Source: CAD feature listing. Evaluate the final solid. Frame: model axes, mm. Face numbers are marked on the shaded views. A direction names the side the tool comes from. Give positions to 0.01 mm unless a question says otherwise; leave off trailing zeros. Order: outer loops, then holes, each group sorted by start corner. A loop starts at its lowest first (then second) coordinate and runs counter-clockwise, first axis right, second up.
from build123d import *

# Parameters (mm, degrees)
F1_DEPTH = 7.62
F3_R     = 1.651
F4_DEPTH = 25.4
F5_R     = 3.175
F6_DEPTH = 3.81
F7_W     = 55.88
F7_H     = 9.525
F8_DEPTH = 2.54


with BuildPart() as f1:
    # F0 (on Right) → F1 (new body, symmetric)
    with BuildSketch(Plane.YZ):
        Polygon((0, 0), (0, -9.8425), (27.94, -9.8425), (27.94, 9.525), (20.447, 9.525), (20.447, 0), align=None)
    extrude(amount=F1_DEPTH, both=True)

    # F2: F1 across plane


with BuildPart() as f1_1:
    add(f1.part)
    add(f1.part.mirror(Plane.XZ))

    # F3 (on face) → F4 (cut)
    with BuildSketch(Plane.YZ.offset(7.62)):
        with Locations((-24.257, 4.445)):
            Circle(F3_R)
        with Locations((24.257, 4.445)):
            Circle(F3_R)
    extrude(amount=-F4_DEPTH, mode=Mode.SUBTRACT)

    # F5 (on face) → F6 (cut)
    with BuildSketch(Plane(origin=(0, 0, -9.8425), x_dir=(1, 0, 0), z_dir=(0, 0, -1))):
        Circle(F5_R)
    extrude(amount=-F6_DEPTH, mode=Mode.SUBTRACT)

    # F7 (on face) → F8 (cut)
    with BuildSketch(Plane.YZ.offset(7.62)):
        with Locations((0, 4.7625)):
            Rectangle(F7_W, F7_H)
    extrude(amount=-F8_DEPTH, mode=Mode.SUBTRACT)


solid = f1_1.part
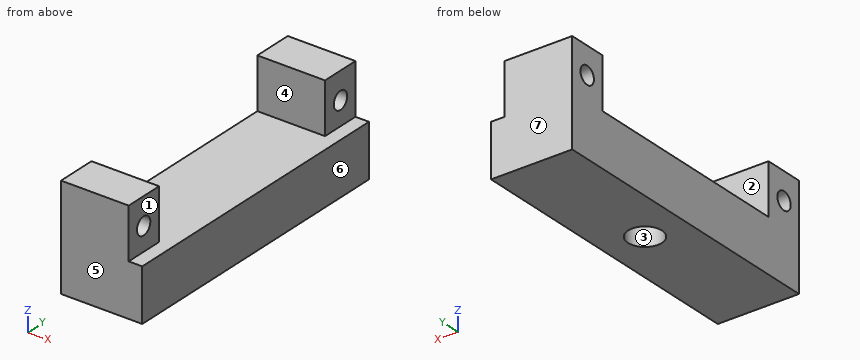
1) Ray query, L1, parallel to X at y = 0, z = -7.4 (3 decimals); L2, parallel to Y at x = -0.5, z = 7.5; L3, parallel to Y at x = -4, z = 3. Return the intervals inside material, ascending.
Checks:
L1: x = -7.62 to -3.175, 3.175 to 7.62
L2: y = -27.94 to -20.45, 20.45 to 27.94
L3: y = -27.94 to -25.06, -23.46 to -20.45, 20.45 to 23.46, 25.06 to 27.94
2) First-contact query: pin 1 Ø5 at (x, y) = (0, -0.5) entering from -Z; pin 2 Ø6 at (y, z) = (-25.5, 6) entering from +X; pin 3 Ø3 at (x, y) = (-0.5, 11.5) entering from +Z. Flat tips, straight axial feed; report the tip coordinate or a pass-through.
Checks:
pin 1: stops at z = -6.03
pin 2: stops at x = 5.08
pin 3: stops at z = 0
3) Section query C-C on y = 0. Output: boundary loops of the cut face in (x, z) (1 decimal).
Checks:
outline: (-7.6, -9.8) - (-3.2, -9.8) - (-3.2, -6) - (3.2, -6) - (3.2, -9.8) - (7.6, -9.8) - (7.6, 0) - (-7.6, 0) - close
4) Pull-direction query (Y, two-part tool) for the marked faces 4, 5, 6 and 7; classes: +Y half, -Y half, draft (parallel to the pull), parting line (faces both ways), or undercut.
Checks:
face 4: undercut
face 5: -Y half
face 6: draft
face 7: +Y half
5) Section query D-D on z = 3.75. Output: boundary loops of the cut face in (x, y), and give its area (3 significant figures).
Checks:
outline: (-7.62, -27.94) - (5.08, -27.94) - (5.08, -25.75) - (-7.62, -25.75) - close; (-7.62, -22.76) - (5.08, -22.76) - (5.08, -20.45) - (-7.62, -20.45) - close; (-7.62, 20.45) - (5.08, 20.45) - (5.08, 22.76) - (-7.62, 22.76) - close; (-7.62, 25.75) - (5.08, 25.75) - (5.08, 27.94) - (-7.62, 27.94) - close
area: 114 mm2
6) Reachability of the marked faces 1, 2 and 3 from +Z, -Z, +X, -X, +Y, -Y: full face, straight path, thin tool, end or side. Return the list, or none.
Checks:
face 1: +Z, +X, +Y, -Y
face 2: +Z, +X, -X
face 3: -Z
7) Section query A-A on z = 1. Output: boundary loops of the cut face in (x, y).
Checks:
outline: (-7.62, -27.94) - (5.08, -27.94) - (5.08, -20.45) - (-7.62, -20.45) - close; (-7.62, 20.45) - (5.08, 20.45) - (5.08, 27.94) - (-7.62, 27.94) - close
8) Section query B-B on x = 0.5. Output: boundary loops of the cut face in (y, z) (1 decimal).
Checks:
outline: (-27.9, -9.8) - (-3.1, -9.8) - (-3.1, -6) - (3.1, -6) - (3.1, -9.8) - (27.9, -9.8) - (27.9, 9.5) - (20.4, 9.5) - (20.4, 0) - (-20.4, 0) - (-20.4, 9.5) - (-27.9, 9.5) - close; hole circle Ø3.3 at (-24.3, 4.4); hole circle Ø3.3 at (24.3, 4.4)
